CAD build for the part. Positions are in the model's coordinates, mm. Round coordinates to 2 decimals unless told otherwise and drop trailing zeros. Write each loop counter-clockwise with the first axis right and the second up, starting at its lowest first coordinate (ties: lowest second). Pieces come first, ordered by that corner, then holes. Notation, with made-up numbers: (83.25, 76.5) -> (96.25, 76.5) arc R7 ccw to (96.25, 89.5) -> close; hole circle Ø11 at (41.5, 38.25). An arc over 180 degrees is marked (long way). Put each result on its own line as item: value. Start each with the question number.
1. Saw through at A-A on x = -105. List the corners of the cut face in (y, z), and give its area (3 significant figures).
2. Saw through at B-B on y = 1. State how many separate pieces and enclosed holes the cut face has, and give its area (3 significant figures).
3. Saw through at C-C on x = -76.5. List the corners of the cut face in (y, z), and give its area (3 significant figures).
4. Saw through at D-D on z = 33. List the corners of the cut face in (x, y).
5. Flat gauge pins, fed straight in: P1, Ø3, axis at y = 2.5, z = -109.5, coming from the +X side; P2, Ø2, axis at x = 28.5, y = 2, coming from the -Z side. Where does each tip first touch, or does it go through?
6. Pull direction X, two halves, no side cores. Call faces 1 (the cylindrical face through (-11.059, 3.219, -27.995)), 2 (the flat face through (-10, 6.35, -63)), 3 (the cylindrical face through (-49.6, 3.13, -125.56)): pulls with the +X half, pulls with the -X half, needs draft (parallel to the pull), parting line crosses it, or undercut.
7. Drill centre lines: line 1 (X direction, y = 2.25, z = 0); line 2 (X direction, y = 1.75, z = -15.5); line 3 (X direction, y = 4.75, z = -14). Where is each one in solid material? Low to high. Write a range as from..to.
from build123d import *

# Parameters (mm, degrees)
SKETCH1_R           = 135
BOSS_EXTRUDE1_DEPTH = 6.35
SKETCH2_R           = 30.1625
CUT_EXTRUDE1_DEPTH  = 192.024402891
SKETCH3_R           = 4.7625
CUT_EXTRUDE2_DEPTH  = 192.024402891


with BuildPart() as part:
    # Sketch1 → Boss-Extrude1 (new body)
    with BuildSketch(Plane(origin=(0, 0, 0), x_dir=(1, 0, 0), z_dir=(0, 1, 0))):
        with Locations(Location((0, 0, 0), (0, 0, 270))):
            Circle(SKETCH1_R)
    extrude(amount=BOSS_EXTRUDE1_DEPTH)

    # Sketch2 → Cut-Extrude1 (cut, through all)
    with BuildSketch(Plane(origin=(0, 6.35, 0), x_dir=(1, 0, 0), z_dir=(0, 1, 0))):
        with BuildLine():
            ThreePointArc((-30.1, 0), (-82.55, -52.45), (-135, 0))
            ThreePointArc((-135, 0), (0, -135), (135, 0))
            ThreePointArc((135, 0), (124.723736889, 51.662263369), (95.45941546, 95.45941546))
            ThreePointArc((95.45941546, 95.45941546), (95.45941546, 21.283914114), (21.283914114, 21.283914114))
            ThreePointArc((21.283914114, 21.283914114), (-11.518771314, 27.808773929), (-30.1, 0))
        make_face()
        with Locations(Location((-82.55, 0, 0), (0, 0, 270))):
            Circle(SKETCH2_R)
    extrude(amount=-CUT_EXTRUDE1_DEPTH, mode=Mode.SUBTRACT)

    # Sketch3 → Cut-Extrude2 (cut, through all)
    with BuildSketch(Plane(origin=(0, 6.35, 0), x_dir=(1, 0, 0), z_dir=(0, 1, 0))):
        with Locations(Location((58.371664787, 58.371664787, 0), (0, 0, 270))):
            Circle(SKETCH3_R)
    extrude(amount=-CUT_EXTRUDE2_DEPTH, mode=Mode.SUBTRACT)


solid = part.part
Return value:
1. outline: (0, -84.85) -> (6.35, -84.85) -> (6.35, -20.14) -> (0, -20.14) -> close; (0, 20.14) -> (6.35, 20.14) -> (6.35, 47.4) -> (0, 47.4) -> close
1. area: 584 mm^2
2. separate pieces: 1
2. enclosed holes: 2
2. area: 26,100 mm^2
3. outline: (0, -111.23) -> (6.35, -111.23) -> (6.35, -29.55) -> (0, -29.55) -> close; (0, 29.55) -> (6.35, 29.55) -> (6.35, 52.1) -> (0, 52.1) -> close
3. area: 662 mm^2
4. outline: (-123.32, 0) -> (-41.78, 0) -> (-41.78, 6.35) -> (-123.32, 6.35) -> close
5. P1: stops at x = 81
5. P2: stops at z = -132.17
6. face 1: undercut
6. face 2: needs draft
6. face 3: parting line crosses it
7. line 1: x = -135..-112.71, -52.39..-30.1
7. line 2: x = -134.11..-108.43, -56.67..-25.8, 28.16..88.59
7. line 3: x = -134.27..-109.27, -55.83..-26.65, 30.4..86.34
